Geometry: final body of the model. Coordinates: model frame, mm. Round coordinates to 2 decimals unless told otherwise and drop trailing zeros. Write each loop counter-clockwise with the first axis right and the second up, starting at its lowest first coordinate (ties: lowest second). Pieces come first, ordered by that corner, then holes. Notation, with made-up numbers: (-4, -28) - (4, -28) arc R18 cw to (4, 2) - close; hole circle Ø11 at (42.25, 33). An arc over 180 degrees is marked (long way). Use a Markdown table: item, result. Add a question column.
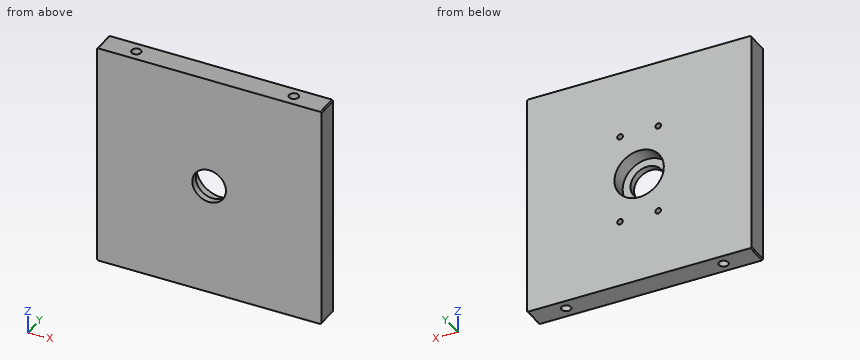
```python
from build123d import *

# Parameters (mm, degrees)
BOSS_EXTRUDE1_DEPTH                  = 5
BOSS_EXTRUDE1_DEPTH_BACK             = 5
SKETCH1_W                            = 100
SKETCH1_H                            = 100
SKETCH1_R                            = 7.5
SKETCH2_R                            = 11
CUT_EXTRUDE1_DEPTH                   = 7
TAP_DRILL_FOR_M5X0_8_TAP1_AT_2_COUNT = 2
TAP_DRILL_FOR_M5X0_8_TAP1_AT_2_PITCH = 70.000402901
TAP_DRILL_FOR_M3X0_5_TAP2_D          = 2.5
TAP_DRILL_FOR_M3X0_5_TAP2_DEPTH      = 6
TAP_DRILL_FOR_M3X0_5_TAP2_TIP        = 0.751075774
CHAMFER1_SIZE                        = 0.5


with BuildPart() as part:
    # Sketch1 → Boss-Extrude1 (new, two sides: drawn at the far end of the back side and taken through both)
    with BuildSketch(Plane(origin=(0, 0, 0), x_dir=(1, 0, 0), z_dir=(0, 1, 0)).offset(-BOSS_EXTRUDE1_DEPTH_BACK)):
        Rectangle(SKETCH1_W, SKETCH1_H)
        with Locations(Location((0, 0, 0), (0, 0, 270))):
            Circle(SKETCH1_R, mode=Mode.SUBTRACT)
    extrude(amount=BOSS_EXTRUDE1_DEPTH + BOSS_EXTRUDE1_DEPTH_BACK)

    # Sketch2 → Cut-Extrude1 (cut)
    with BuildSketch(Plane(origin=(0, 5, 0), x_dir=(1, 0, 0), z_dir=(0, 1, 0))):
        with Locations(Location((0, 0, 0), (0, 0, 270))):
            Circle(SKETCH2_R)
    extrude(amount=-CUT_EXTRUDE1_DEPTH, mode=Mode.SUBTRACT)

    # Sketch6 → Tap Drill for M5x0.8 Tap1 (revolve, cut)
    with BuildSketch(Plane(origin=(-35, 0, 50), x_dir=(0, -1, 0), z_dir=(1, 0, 0))):
        Polygon((0, 0), (0, 11.2618073), (2.1, 10), (2.1, 0), align=None)
    tap_drill_for_m5x0_8_tap1 = revolve(axis=Axis((-35, 0, 56.35), (0, 0, -1)), mode=Mode.SUBTRACT)

    # Tap Drill for M5x0.8 Tap1 at 2: Tap Drill for M5x0.8 Tap1 ×2
    with Locations(*[Vector(0.9999942443098965, 0.0033928376146228614, 0) * (i * TAP_DRILL_FOR_M5X0_8_TAP1_AT_2_PITCH) for i in range(1, TAP_DRILL_FOR_M5X0_8_TAP1_AT_2_COUNT)]):
        add(tap_drill_for_m5x0_8_tap1, mode=Mode.SUBTRACT)

    # Mirror1: Tap Drill for M5x0.8 Tap1 across plane
    add(tap_drill_for_m5x0_8_tap1.mirror(Plane(origin=(0, 0, 0), x_dir=(1, 0, 0), z_dir=(0, 0, -1))), mode=Mode.SUBTRACT)

    # Mirror1 copy 1 sketch → Mirror1 copy 1 (revolve, cut)
    with BuildSketch(Plane(origin=(35, 0.2375, -50), x_dir=(0, -1, 0), z_dir=(1, 0, 0))):
        Polygon((0, 0), (0, -11.2618073), (2.1, -10), (2.1, 0), align=None)
    revolve(axis=Axis((35, 0.2375, -56.35), (0, 0, -1)), mode=Mode.SUBTRACT)

    # Tap Drill for M3x0.5 Tap2
    with Locations(Plane(origin=(0, 5, 0), x_dir=(1, 0, 0), z_dir=(0, 1, 0))):
        with Locations((-8.5, -20), (8.5, -20), (8.5, 20), (-8.5, 20)):
            Hole(TAP_DRILL_FOR_M3X0_5_TAP2_D / 2, depth=TAP_DRILL_FOR_M3X0_5_TAP2_DEPTH)
            with Locations((0, 0, -(TAP_DRILL_FOR_M3X0_5_TAP2_DEPTH + TAP_DRILL_FOR_M3X0_5_TAP2_TIP / 2))):  # 118° drill point
                Cone(0, TAP_DRILL_FOR_M3X0_5_TAP2_D / 2, TAP_DRILL_FOR_M3X0_5_TAP2_TIP, mode=Mode.SUBTRACT)

    # Chamfer1
    chamfer1_edges = [part.edges().sort_by_distance(p)[0] for p in [
        (-50, 0, -50),
        (50, 0, -50),
        (50, 0, 50),
        (-50, 0, 50),
    ]]
    chamfer(chamfer1_edges, length=CHAMFER1_SIZE)


solid = part.part
```
1) Pin query (flat end, axial travel): P1, Ø2, axis at x = -8.5, z = -20, coming from the +Y side; P2, Ø4, axis at x = -35, y = 0, coming from the -Z side; P3, Ø3.5, axis at x = 35, y = 0.24, coming from the -Z side; P4, Ø17.5, axis at x = -4.5, z = 1, coming from the +Y side. Return the tip coordinate at first contact, or that it passes through.
2) Section B-B, the plane z = -5.5. Return the cut outline in (x, y), then the cut area to 3 significant figures.
3) Material intervals for L1, parallel to X at y = 2.2, z = -20; L2, parallel to X at y = 0, z = 47.5; L3, parallel to Y at x = -35, z = -47.25, sorted ascending. Write a range as from..to.
4) Section A-A, the plane x = 0. Return the cut outline in (y, z), then the cut area to 3 significant figures.
Output values:
| question | item | result |
|---|---|---|
| 1 | P1 | stops at y = -1.15 |
| 1 | P2 | stops at z = -39.94 |
| 1 | P3 | stops at z = -39.79 |
| 1 | P4 | stops at y = 5 |
| 2 | outline | (-50, -5) - (-5.1, -5) - (-5.1, -2) - (-9.53, -2) - (-9.53, 5) - (-50, 5) - close; (5.1, -5) - (50, -5) - (50, 5) - (9.53, 5) - (9.53, -2) - (5.1, -2) - close |
| 2 | area | 836 mm^2 |
| 3 | L1 | x = -50..-9.75, -7.25..7.25, 9.75..50 |
| 3 | L2 | x = -50..-37.1, -32.9..32.91, 37.09..50 |
| 3 | L3 | y = -5..-2.1, 2.1..5 |
| 4 | outline | (-5, -50) - (5, -50) - (5, -11) - (-2, -11) - (-2, -7.5) - (-5, -7.5) - close; (-5, 7.5) - (-2, 7.5) - (-2, 11) - (5, 11) - (5, 50) - (-5, 50) - close |
| 4 | area | 801 mm^2 |
